from build123d import *

# Parameters (mm, degrees)
SKETCH_1_R          = 4
EXTRUDE_1_DEPTH     = 2
SKETCH_2_R          = 1.5
CUT_EXTRUDE_1_DEPTH = 7
CHAMFER_1_SIZE      = 1.5
CHAMFER_2_SIZE      = 0.5


with BuildPart() as part:
    # 草图1 → 凸台-拉伸1 (new body)
    with BuildSketch(Plane(origin=(0, 0, 0), x_dir=(1, 0, 0), z_dir=(0, 1, 0))):
        with Locations(Location((0, 0, 0), (0, 0, 270))):
            Circle(SKETCH_1_R)
    extrude(amount=EXTRUDE_1_DEPTH)

    # 草图2 → 切除-拉伸1 (cut, through all)
    with BuildSketch(Plane(origin=(0, 2, 0), x_dir=(1, 0, 0), z_dir=(0, 1, 0))):
        with Locations(Location((0, 0, 0), (0, 0, 270))):
            Circle(SKETCH_2_R)
    extrude(amount=-CUT_EXTRUDE_1_DEPTH, mode=Mode.SUBTRACT)

    # 倒角1
    chamfer_1_edges = [part.edges().sort_by_distance(p)[0] for p in [
        (0, 2, -1.5),
    ]]
    chamfer(chamfer_1_edges, length=CHAMFER_1_SIZE)

    # 倒角2
    chamfer_2_edges = [part.edges().sort_by_distance(p)[0] for p in [
        (0, 2, -3),
        (0, 2, -4),
    ]]
    chamfer(chamfer_2_edges, length=CHAMFER_2_SIZE - 0.0001)  # a hair under: the kernel refuses the full size


solid = part.part
Part model, mm, in its own coordinate system. Coordinates: 2 decimals unless noted, no trailing zeros. Order: outer loops, then holes, each group sorted by start corner. A loop starts at its lowest first (then second) coordinate and runs counter-clockwise, first axis right, second up. Notation, with made-up numbers: M 48.25,4 L 90.25,4 A7 ccw 90.25,10 Z; hole C 8,85.5 d4. An arc over 180 degrees is marked long. Use a Markdown table: item, result.
(1) Cut at C-C on y = 1. Write the cut outline in (x, z).
A:
| item | result |
|---|---|
| outline | C 0,0 d8; hole C 0,0 d4 |
(2) Probe L1, parallel to X at y = 0.4, z = 0; L2, parallel to Z at x = 3, y = 0.75; L3, parallel to Y at x = 1.5, z = 2. List the from-to ranges inside material, lowest first.
A:
| item | result |
|---|---|
| L1 | x = -4 to -1.5, 1.5 to 4 |
| L2 | z = -2.65 to 2.65 |
| L3 | y = 0 to 1.5 |
(3) Pull direction Z, two halves, no side cores. Call faces 1 (the flat face through (0, 0, 2)), 2 (the cylindrical face through (-3.905, 0.74, -0.867)), 3 (the cylindrical face through (0.45, 0.25, 1.43)): released by +Z, released by -Z, zero draft, split by the parting line, or undercut.
A:
| item | result |
|---|---|
| face 1 | zero draft |
| face 2 | split by the parting line |
| face 3 | undercut |
(4) Flat gauge pin, fed straight in: pin 1 (1 mm diameter, centred on y = 0.5, z = -2, fed in from -X). Where does the tip first touch, or does it go through?
A:
| item | result |
|---|---|
| pin 1 | stops at x = -3.71 |
